Can you work these out from the drawing? Everything is in mm from the part's minimum corner. A direction names the side the tool comes from. Round coordinates to 2 decimals unless told otherwise and drop trailing zeros. Order: outer loops, then holes, each group sorted by start corner. A loop starts at its lowest first (then second) coordinate and runs counter-clockwise, first axis right, second up. Notation, with made-up numbers: (38, 16.5) -> (80, 16.5) arc R26 ccw to (80, 47.5) -> close; hole circle Ø11 at (84.25, -35). An arc over 180 degrees is marked (long way). One line per item, written item: value.
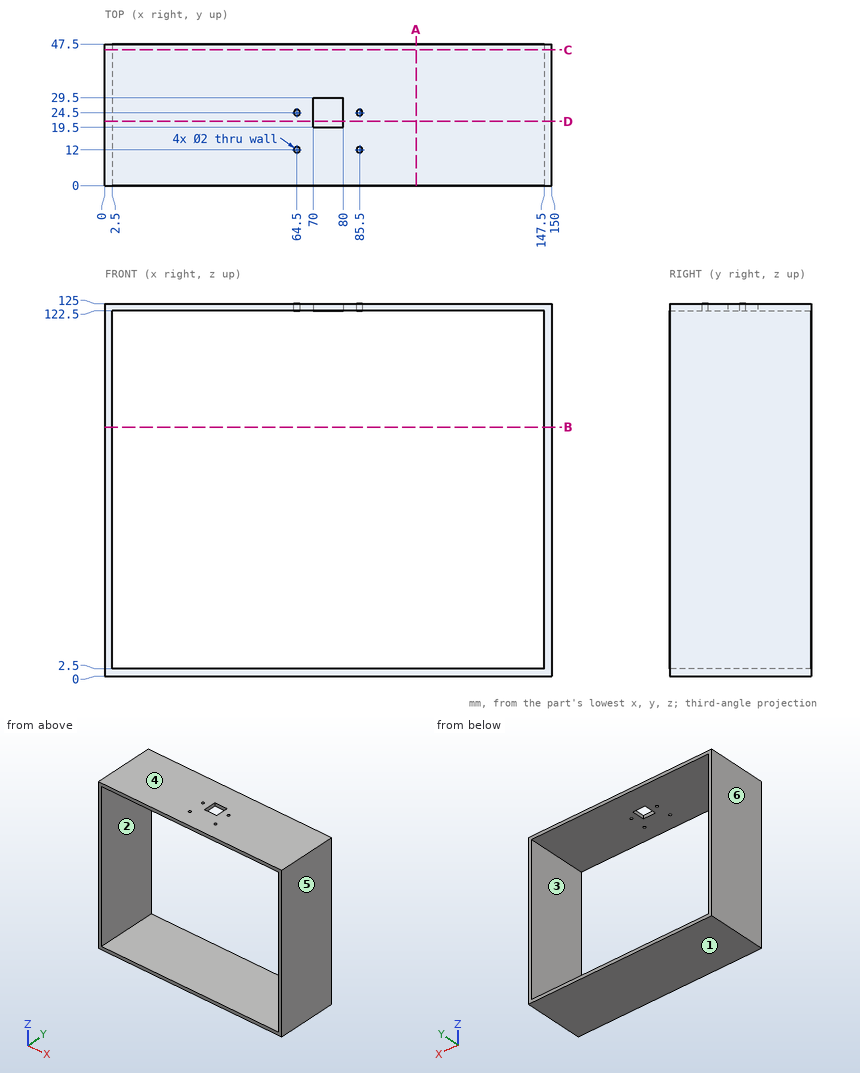
Q1. We'd pull the mould along X, two halves only. Please class the marked faces 3, 4, 5 and 6: released by +X, released by -X, zero draft, split by the parting line, or undercut.
Answers below:
face 3: undercut
face 4: zero draft
face 5: released by +X
face 6: released by -X
Q2. I want a section at D-D on y = 21.5. List the corners of the cut face in (x, z) for me.
Answers below:
outline: (0, 0) -> (150, 0) -> (150, 125) -> (80, 125) -> (80, 122.5) -> (147.5, 122.5) -> (147.5, 2.5) -> (2.5, 2.5) -> (2.5, 122.5) -> (70, 122.5) -> (70, 125) -> (0, 125) -> close
Q3. Will this pin go through, and if not, where does the flat tip stop? pin 1 Ø1.2 at (x, y) = (64.5, 12) entering from +Z.
Answers below:
pin 1: z = 2.5
Q4. I want a section at A-A on x = 104.5. List the corners of the cut face in (y, z) for me, plus the area to 4 significant figures.
Answers below:
outline: (0, 0) -> (47.5, 0) -> (47.5, 2.5) -> (0, 2.5) -> close; (0, 122.5) -> (47.5, 122.5) -> (47.5, 125) -> (0, 125) -> close
area: 237.5 mm^2
Q5. I want a section at B-B on z = 83.5. List the corners of the cut face in (x, y) for me.
Answers below:
outline: (0, 0) -> (2.5, 0) -> (2.5, 47.5) -> (0, 47.5) -> close; (147.5, 0) -> (150, 0) -> (150, 47.5) -> (147.5, 47.5) -> close
Q6. Please list where these lines run through material, in increasing order: line 1 along X through (y, z) = (41.5, 44); line 2 along Z through (x, y) = (120, 15.5); line 3 along Y through (x, z) = (64.5, 123.1).
Answers below:
line 1: 0 to 2.5, 147.5 to 150
line 2: 0 to 2.5, 122.5 to 125
line 3: 0 to 11, 13 to 23.5, 25.5 to 47.5
Q7. I want a section at C-C on y = 45.5. List the corners of the cut face in (x, z) for me.
Answers below:
outline: (0, 0) -> (150, 0) -> (150, 125) -> (0, 125) -> close; hole (2.5, 2.5) -> (147.5, 2.5) -> (147.5, 122.5) -> (2.5, 122.5) -> close
Q8. On a 3-axis mill with a long thin cutter (end or side, diameter ignored), from which of +Z, -Z, +X, -X, +Y, -Y can I reach the whole of each face in a straight line? I mean the marked faces 1 and 2. Say none if no direction works.
Answers below:
face 1: -Z, +X, -X, +Y, -Y
face 2: +Y, -Y
